The model under review builds one solid part; all positions refer to its coordinate system, in mm. Give positions to 0.01 mm unless a question says otherwise; leave off trailing zeros. Order: outer loops, then holes, each group sorted by start corner. A loop starts at its lowest first (then second) coordinate and runs counter-clockwise, first axis right, second up. Notation, with made-up numbers: (70, 41.5) -> (100, 41.5) arc R18 cw to (100, 64.5) -> close; hole circle Ø4 at (11.5, 16.5). An arc over 180 degrees is marked (long way). Answer as a JSON object with one key per item and string values. Group by question number.
from build123d import *

# Parameters (mm, degrees)
SKETCH_1_R          = 180
EXTRUDE_1_DEPTH     = 20
SKETCH_3_R          = 40
CUT_EXTRUDE_2_DEPTH = 254
CUT_EXTRUDE_3_REACH = 257.343


with BuildPart() as part:
    # 草图1 → 凸台-拉伸1 (new body)
    with BuildSketch(Plane.XY):
        Circle(SKETCH_1_R)
    extrude(amount=EXTRUDE_1_DEPTH)

    # 草图3 → 切除-拉伸2 (cut)
    with BuildSketch(Plane.XY.offset(20)):
        Circle(SKETCH_3_R)
    extrude(amount=-CUT_EXTRUDE_2_DEPTH, mode=Mode.SUBTRACT)

    # 草图2 → 切除-拉伸3 (cut, up to next)
    with BuildSketch(Plane.XY.offset(20), mode=Mode.PRIVATE) as cut_extrude_3_sk1:
        with BuildLine():
            Line((-110, 34), (-150, 34))
            ThreePointArc((-150, 34), (-154, 30), (-150, 26))
            Line((-150, 26), (-110, 26))
            ThreePointArc((-110, 26), (-106, 30), (-110, 34))
        make_face()
    cut_extrude_3_tool1 = extrude(cut_extrude_3_sk1.sketch, amount=-CUT_EXTRUDE_3_REACH, mode=Mode.PRIVATE) & part.part
    # 草图2 → 切除-拉伸3 (cut, up to next)
    with BuildSketch(Plane.XY.offset(20), mode=Mode.PRIVATE) as cut_extrude_3_sk2:
        with BuildLine():
            Line((-110, -34), (-150, -34))
            ThreePointArc((-150, -34), (-154, -30), (-150, -26))
            Line((-150, -26), (-110, -26))
            ThreePointArc((-110, -26), (-106, -30), (-110, -34))
        make_face()
    cut_extrude_3_tool2 = extrude(cut_extrude_3_sk2.sketch, amount=-CUT_EXTRUDE_3_REACH, mode=Mode.PRIVATE) & part.part
    # 草图2 → 切除-拉伸3 (cut, up to next)
    with BuildSketch(Plane.XY.offset(20), mode=Mode.PRIVATE) as cut_extrude_3_sk3:
        with BuildLine():
            Line((110, 34), (150, 34))
            ThreePointArc((150, 34), (154, 30), (150, 26))
            Line((150, 26), (110, 26))
            ThreePointArc((110, 26), (106, 30), (110, 34))
        make_face()
    cut_extrude_3_tool3 = extrude(cut_extrude_3_sk3.sketch, amount=-CUT_EXTRUDE_3_REACH, mode=Mode.PRIVATE) & part.part
    # 草图2 → 切除-拉伸3 (cut, up to next)
    with BuildSketch(Plane.XY.offset(20), mode=Mode.PRIVATE) as cut_extrude_3_sk4:
        with BuildLine():
            Line((110, -34), (150, -34))
            ThreePointArc((150, -34), (154, -30), (150, -26))
            Line((150, -26), (110, -26))
            ThreePointArc((110, -26), (106, -30), (110, -34))
        make_face()
    cut_extrude_3_tool4 = extrude(cut_extrude_3_sk4.sketch, amount=-CUT_EXTRUDE_3_REACH, mode=Mode.PRIVATE) & part.part
    add(cut_extrude_3_tool1.solids().sort_by_distance((-130, 30, 20))[0], mode=Mode.SUBTRACT)
    add(cut_extrude_3_tool2.solids().sort_by_distance((-130, -30, 20))[0], mode=Mode.SUBTRACT)
    add(cut_extrude_3_tool3.solids().sort_by_distance((130, 30, 20))[0], mode=Mode.SUBTRACT)
    add(cut_extrude_3_tool4.solids().sort_by_distance((130, -30, 20))[0], mode=Mode.SUBTRACT)


solid = part.part
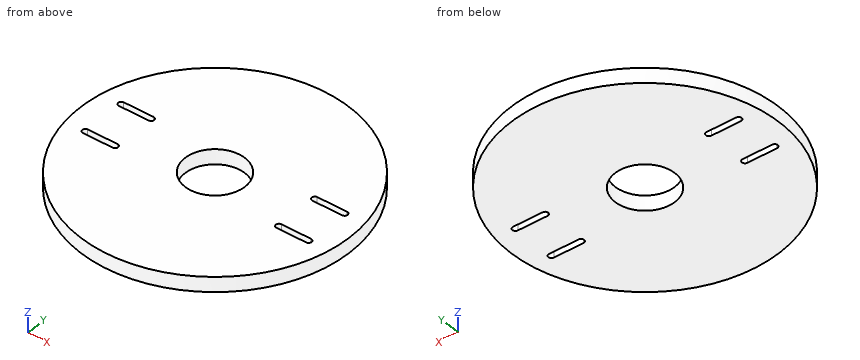
1. Take a section at C-C on y = -12. Give the boundary of the cut face in (x, z).
2. Take a section at A-A on z = 4. Give the boundary of the cut face in (x, y).
3. For pin 1 (10 mm diameter, centred on x = 77, y = 5, fed in from -Z); pin 2 (6 mm diameter, centred on x = -123, z = 11, fed in from +Y); pin 3 (10 mm diameter, centred on x = 133.5, z = 10, fed in from -Y); pin 4 (2 mm diameter, centred on y = 126, z = 10.5, fed in from -X), all flat-tipped, find the tip position at first contact; note any pin that passes through.
4. Take a section at D-D on y = 64. Give the boundary of the cut face in (x, z).
5. Take a section at B-B on x = 8.5. Give the boundary of the cut face in (y, z), plus the area to 3 significant figures.
6. For probe 1 along Y at (x, z) = (-118.5, 6); probe 2 along Y at (x, z) = (-133.5, 12.5); probe 3 along Y at (x, z) = (0, 11.5), list the stretches that pass through material, from the lowest coordinate up. Write a range as [from, to].
Checks:
{
 "1": {"outline": "(-179.6, 0) -> (-38.16, 0) -> (-38.16, 20) -> (-179.6, 20) -> close; (38.16, 0) -> (179.6, 0) -> (179.6, 20) -> (38.16, 20) -> close"},
 "2": {"outline": "circle Ø360 at (0, 0); hole (-150, -34) -> (-110, -34) arc R4 ccw to (-110, -26) -> (-150, -26) arc R4 ccw to start; hole (-150, 26) -> (-110, 26) arc R4 ccw to (-110, 34) -> (-150, 34) arc R4 ccw to start; hole circle Ø80 at (0, 0); hole (110, -34) -> (150, -34) arc R4 ccw to (150, -26) -> (110, -26) arc R4 ccw to start; hole (110, 26) -> (150, 26) arc R4 ccw to (150, 34) -> (110, 34) arc R4 ccw to start"},
 "3": {"pin 1": "stops at z = 0", "pin 2": "stops at y = 134.16", "pin 3": "stops at y = -126.05", "pin 4": "stops at x = -129.52"},
 "4": {"outline": "(-168.24, 0) -> (168.24, 0) -> (168.24, 20) -> (-168.24, 20) -> close"},
 "5": {"outline": "(-179.8, 0) -> (-39.09, 0) -> (-39.09, 20) -> (-179.8, 20) -> close; (39.09, 0) -> (179.8, 0) -> (179.8, 20) -> (39.09, 20) -> close", "area": "5,630 mm2"},
 "6": {"probe 1": "y = [-135.49, -34], [-26, 26], [34, 135.49]", "probe 2": "y = [-120.74, -34], [-26, 26], [34, 120.74]", "probe 3": "y = [-180, -40], [40, 180]"}
}
